The listing builds one solid part. Answer for the finished solid, in the listing's coordinates (mm). Round coordinates to 2 decimals unless told otherwise and drop trailing zeros. Write each loop counter-clockwise with the first axis right and the second up, starting at its lowest first coordinate (ties: lowest second). Pieces come first, ordered by that corner, then holes. Notation, with made-up numbers: (18, 44) - (55, 44) arc R31 cw to (55, 72) - close; hole circle Ø4 at (-30, 72). An arc over 180 degrees is marked (long way). Answer in a Markdown table with one row per item.
Autodesk Inventor part; units mm, degrees
ref_plane "YZ Plane" through (0, 0, 0) normal (1, 0, 0) x (0, 1, 0)
ref_plane "XZ Plane" through (0, 0, 0) normal (0, 1, 0) x (-1, 0, 0)
ref_plane "XY Plane" through (0, 0, 0) normal (0, 0, 1) x (1, 0, 0)
sketch "スケッチ1" plane through (0, 0, 0) normal (1, 0, 0) x (0, 1, 0)
  line L0 (-700, 210) -> (-700, 490)
  line L1 (-700, 490) -> (-400, 690)
  line L2 (-400, 690) -> (-250, 690)
  line L3 (-250, 690) -> (0, 150)
  line L4 (0, 150) -> (0, 0)
  line L5 (0, 0) -> (-230, 0)
  arc A0 (-230, 0) -> (-700, 210) centre (-700, -420.9524) ccw
  dimension "d0" = 690
  dimension "d1" = 280
  dimension "d2" = 200
  dimension "d3" = 300
  dimension "d4" = 150
  dimension "d5" = 700
  dimension "d6" = 230
  dimension "d7" = 150
extrude "押し出し1" add sketch "スケッチ1" along normal blind 5
sketch "スケッチ2" plane through (5, 0, 0) normal (1, 0, 0) x (0, 0, -1)
  circle A0 centre (-100, -87) radius 2.5
  line L0 (0, 0) -> (-150, 0)
  line L1 (0, -230) -> (0, 0)
  circle A1 centre (-155, -150) radius 2.5
  dimension "d10" = 87
  dimension "d11" = 100
  dimension "d12" = 5
  dimension "d13" = 150
  dimension "d14" = 155
  dimension "d15" = 5
extrude "押し出し2" cut sketch "スケッチ2" against normal through all
properties part number "end_plate" material "CFRP"
(1) Flat-ended cylindrical pins translate along their axes: pin 1 (4 mm diameter, centred on y = -87, z = 100, fed in from -X); pin 2 (3 mm diameter, centred on x = 3, y = -236, fed in from -Z). Find the tip coordinate at first contact, or state that the pin passes through.
Checked values:
| item | result |
|---|---|
| pin 1 | passes through |
| pin 2 | stops at z = 4.97 |
(2) Section B-B (y = -192.5) is taken. Give the vertices of the cut face in (x, z), and give its area (3 significant figures).
Checked values:
| item | result |
|---|---|
| outline | (0, 0) - (5, 0) - (5, 565.8) - (0, 565.8) - close |
| area | 2,830 mm2 |
(3) Section C-C (y = -69) is taken. Give the vertices of the cut face in (x, z).
Checked values:
| item | result |
|---|---|
| outline | (0, 0) - (5, 0) - (5, 299.04) - (0, 299.04) - close |
(4) Find the intervals of material crossed by line 1 (Y direction, x = 1.3, z = 155); line 2 (Z direction, x = 2.5, y = -150); line 3 (Y direction, x = 1.4, z = 343), in increasing order.
Checked values:
| item | result |
|---|---|
| line 1 | y = -442.36 to -152.5, -147.5 to -2.31 |
| line 2 | z = 0 to 152.5, 157.5 to 474 |
| line 3 | y = -700 to -89.35 |
(5) Section A-A (x = 0.85) is taken. Give the vertices of the cut face in (y, z).
Checked values:
| item | result |
|---|---|
| outline | (-700, 210) arc R630.95 cw to (-230, 0) - (0, 0) - (0, 150) - (-250, 690) - (-400, 690) - (-700, 490) - close; hole circle Ø5 at (-150, 155); hole circle Ø5 at (-87, 100) |
